Answer from the drawing. Dimensions are ordinates in mm from the lowest x, y and z of the part. A direction names the side the tool comes from. Round coordinates to 2 decimals unless told otherwise and drop trailing zeros. Loops run counter-clockwise (first coordinate to the right, second up) from the corner with the lowest first, then second, coordinate; pieces in that order, holes last. Notation, with made-up numbers: (-13, 39) - (35, 39) arc R34 cw to (35, 75) - close; hole circle Ø7 at (6, 24.5). An arc over 180 degrees is marked (long way). Return JSON: item names as keys, results as strings.
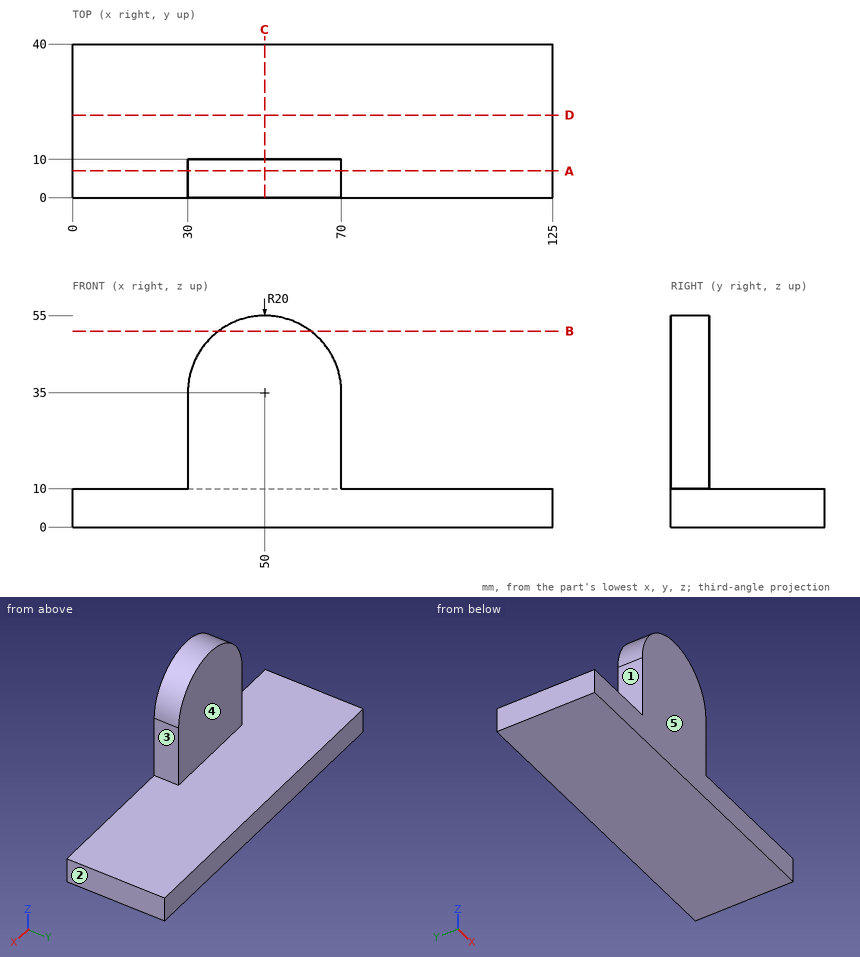
1) A tool of negligible diameter and unlimited length cuts with its end or side. For the marked faces 1, 2, 3, 4 and 5, from which of +Z, -Z, +X, -X, +Y, -Y can it reach the whole face along a straight path? Write none if from no direction.
Verdict:
{"face 1": "+Z, -X, +Y, -Y", "face 2": "+Z, -Z, +X, +Y, -Y", "face 3": "+Z, +X, +Y, -Y", "face 4": "+Z, +X, -X, +Y", "face 5": "+Z, -Z, +X, -X, -Y"}
2) Flat-ended cylindrical pins translate along their axes: pin 1 (6 mm diameter, centred on x = 47.5, z = 23, fed in from +Y); pin 2 (11 mm diameter, centred on y = 4.5, z = 26.5, fed in from -X); pin 3 (12 mm diameter, centred on y = 17.5, z = 29.5, fed in from -X); pin 4 (3 mm diameter, centred on x = 54, y = 15.5, fed in from +Z). Find the tip coordinate at first contact, or state that the pin passes through.
Verdict:
{"pin 1": "stops at y = 10", "pin 2": "stops at x = 30", "pin 3": "passes through", "pin 4": "stops at z = 10"}
3) Section C-C (x = 50) is taken. Give the vertices of the cut face in (y, z).
Verdict:
{"outline": "(0, 0) - (40, 0) - (40, 10) - (10, 10) - (10, 55) - (0, 55) - close"}
4) Section A-A (y = 7) is taken. Give the vertices of the cut face in (x, z).
Verdict:
{"outline": "(0, 0) - (125, 0) - (125, 10) - (70, 10) - (70, 35) arc R20 ccw to (30, 35) - (30, 10) - (0, 10) - close"}
5) Section D-D (y = 21.5) is taken. Give the vertices of the cut face in (x, z), and give its area (3 significant figures).
Verdict:
{"outline": "(0, 0) - (125, 0) - (125, 10) - (0, 10) - close", "area": "1,250 mm2"}
6) Section B-B (z = 51) is taken. Give the vertices of the cut face in (x, y).
Verdict:
{"outline": "(38, 0) - (62, 0) - (62, 10) - (38, 10) - close"}
7) Find the intervals of material crossed by L1, parallel to Y at x = 64.5, z = 17.5, in increasing order.
Verdict:
{"L1": "y = 0 to 10"}
